Geometry: final body of the model. Coordinates: model frame, mm. A direction names the side the tool comes from. Round coordinates to 2 decimals unless told otherwise and drop trailing zeros. Loops run counter-clockwise (first coordinate to the right, second up) from the corner with the lowest first, then second, coordinate; pieces in that order, holes last. Notation, with made-up numbers: M 51,34 L 83,34 A29 ccw 83,55 Z; hole C -11.5,-37.5 d4. An arc over 180 degrees is marked long. Return JSON: item names as keys, results as strings.
from build123d import *

# Parameters (mm, degrees)
F0_W     = 19.05
F0_H     = 76.2
F1_DEPTH = 19.05


with BuildPart() as f1:
    # F0 (on Front) → F1 (new body)
    with BuildSketch(Plane.XZ):
        Polygon((80.788266, 152.4), (-338.311734, 152.4), (-338.311734, -10.011766), (-338.311734, -86.211766), (-338.311734, -162.411766), (-338.311734, -238.611766), (-338.311734, -304.8), (80.788266, -304.8), (80.788266, -228.6), (80.788266, -152.4), (80.788266, -76.2), (80.788266, 0), (80.788266, 76.2), align=None)
        with Locations((-347.836734, -48.111766)):
            Rectangle(F0_W, F0_H)
        with Locations((-347.836734, -200.511766)):
            Rectangle(F0_W, F0_H)
        with Locations((90.313266, -38.1)):
            Rectangle(F0_W, F0_H)
        with Locations((90.313266, -190.5)):
            Rectangle(F0_W, F0_H)
    extrude(amount=F1_DEPTH)


solid = f1.part
Q1. Pull-direction query (Z, two-part tool) for faces 4 (the flat face through (-348, -9, -86.212)), 5 (the flat face through (-348, -9, -238.612)), 6 (the flat face through (-132, -19.05, -73)); classes: pulls with the +Z half, pulls with the -Z half, needs draft (parallel to the pull), parting line crosses it, or undercut.
Determined:
{"face 4": "undercut", "face 5": "pulls with the -Z half", "face 6": "needs draft"}
Q2. Section query B-B (z = -246.5). Output: boundary loops of the cut face in (x, y), plus the area to 3 significant figures.
Determined:
{"outline": "M -338.31,-19.05 L 80.79,-19.05 L 80.79,0 L -338.31,0 Z", "area": "7,980 mm^2"}
Q3. Section query A-A (y = -3.5). Output: boundary loops of the cut face in (x, z), plus the area to 3 significant figures.
Determined:
{"outline": "M -357.36,-238.61 L -338.31,-238.61 L -338.31,-304.8 L 80.79,-304.8 L 80.79,-228.6 L 99.84,-228.6 L 99.84,-152.4 L 80.79,-152.4 L 80.79,-76.2 L 99.84,-76.2 L 99.84,0 L 80.79,0 L 80.79,152.4 L -338.31,152.4 L -338.31,-10.01 L -357.36,-10.01 L -357.36,-86.21 L -338.31,-86.21 L -338.31,-162.41 L -357.36,-162.41 Z", "area": "197,000 mm^2"}
Q4. Material intervals for L1, parallel to X at y = -3.25, z = 2.5; L2, parallel to X at y = -4, z = -81, sorted ascending.
Determined:
{"L1": "x = -338.31 to 80.79", "L2": "x = -357.36 to 80.79"}
Q5. Pin query (flat end, axial travel): pin 1 (4 mm diameter, centred on y = -8.5, z = -156, fed in from -X); pin 2 (5.5 mm diameter, centred on x = 86, y = -14, fed in from -Z); pin 3 (5.5 mm diameter, centred on y = -6, z = 81.5, fed in from +X). Return the tip coordinate at first contact, or that it passes through.
Determined:
{"pin 1": "stops at x = -338.31", "pin 2": "stops at z = -228.6", "pin 3": "stops at x = 80.79"}
Q6. Reachability of faces 1 (the flat face through (90, -9, -76.2)), 2 (the flat face through (80.788, -9, -267)), 3 (the flat face through (-348, -9, -162.412)) from +Z, -Z, +X, -X, +Y, -Y: full face, straight path, thin tool, end or side. Return the list, or none.
Determined:
{"face 1": "+X, +Y, -Y", "face 2": "-Z, +X, +Y, -Y", "face 3": "-X, +Y, -Y"}
